Can you work these out from the model? Positions are in its coordinate system, mm. A direction names the side the tool comes from. Round coordinates to 2 decimals unless told otherwise and drop trailing zeros. Loops run counter-clockwise (first coordinate to the right, second up) from the corner with the lowest first, then second, coordinate; pieces in that order, holes last. Notation, with made-up numbers: M 41.25,-29 L 83.25,-29 A17 cw 83.25,-17 Z; hole C -36.5,33.5 d3. An arc over 180 degrees is marked long. Return JSON: item names as keys, results as strings.
Autodesk Inventor part; units mm, degrees
ref_plane "YZ Plane" through (0, 0, 0) normal (1, 0, 0) x (0, 1, 0)
ref_plane "XZ Plane" through (0, 0, 0) normal (0, 1, 0) x (-1, 0, 0)
ref_plane "XY Plane" through (0, 0, 0) normal (0, 0, 1) x (1, 0, 0)
sketch "Sketch1" plane through (0, 0, 0) normal (0, 0, 1) x (1, 0, 0)
  circle A0 centre (0, 0) radius 7
  line L0 (0, 0) -> (0, -11.43) construction
  line L1 (0, -11.43) -> (-50.8, -11.43) construction
  circle A1 centre (-50.8, -11.43) radius 7
  line L2 (0, -11.43) -> (0, -24.13) construction
  line L3 (-50.8, -11.43) -> (-50.8, -24.13) construction
  line L4 (0, -24.13) -> (-101.6, -24.13) construction
  line L5 (-101.6, -24.13) -> (-101.6, -125.73) construction
  line L6 (0, -24.13) -> (12.7, -24.13) construction
  line L7 (-101.6, -125.73) -> (-35.3, -24.13) construction
  line L8 (-101.6, -125.73) -> (15.6852, -125.73) construction
  line L9 (-35.3, -24.13) -> (-117.1955, 29.3117) construction
  line L10 (-117.1955, 29.3117) -> (-143.4272, -10.8866) construction
  line L11 (-123.0577, 33.1371) -> (-149.2895, -7.0611) construction
  line L12 (-137.565, -14.712) -> (-111.3333, 25.4862) construction
  arc A2 (-111.3333, 25.4862) -> (-123.0577, 33.1371) centre (-117.1955, 29.3117) ccw construction
  arc A3 (-149.2895, -7.0611) -> (-137.565, -14.712) centre (-143.4272, -10.8866) ccw construction
  circle A4 centre (-117.1955, 29.3117) radius 12.7 construction
  circle A5 centre (0, 0) radius 120.8055 construction
  circle A6 centre (-50.8, -11.43) radius 92.6288 construction
  line L13 (-101.6, -125.73) -> (-152.4, -125.73) construction
  line L14 (-152.4, -125.73) -> (-152.4, -87.63) construction
  circle A7 centre (-152.4, -87.63) radius 38.1
  line L15 (-152.4, -87.63) -> (-152.4, -49.53) construction
  line L16 (-152.4, -49.53) -> (-152.4, -36.83) construction
  circle A8 centre (-152.4, -36.83) radius 12.7 construction
  circle A9 centre (-117.1955, 29.3117) radius 10.16
  circle A10 centre (-152.4, -36.83) radius 12.7
  line L17 (-163.4022, -30.4863) -> (-125.9972, 34.3866)
  line L18 (-152.4, -49.53) -> (-117.1955, -49.53)
  circle A11 centre (-130.3114, 9.2125) radius 2.05
  circle A12 centre (-143.4272, -10.8866) radius 2.05
  circle A13 centre (-117.1955, 29.3117) radius 7
  circle A14 centre (-152.4, -36.83) radius 7
  line L19 (-117.1955, -49.53) -> (-107.1202, 28.0024)
  point P0 (-152.4, -49.53)
  dimension "d0" = 14
  dimension "d1" = 11.43
  dimension "d2" = 50.8
  dimension "d3" = 14
  dimension "d4" = 12.7
  dimension "d5" = 12.7
  dimension "d6" = 101.6
  dimension "d7" = 101.6
  dimension "d8" = 12.7
  dimension "d9" = 48
  dimension "d14" = 97.79
  dimension "d15" = 90
  dimension "d16" = 48
  dimension "d17" = 14
  dimension "d18" = 25.4
  dimension "d19" = 50.8
  dimension "d20" = 38.1
  dimension "d21" = 12.7
  dimension "d22" = 20.32
  dimension "d24" = 4.1
  dimension "d25" = 4.1
  dimension "d26" = 14
extrude "Extrusion1" add sketch "Sketch1" along normal blind 6.35 contours A10 | A10 L17 A9 L19 L18 | A9
fillet "Fillet1" radius 6.35 1 edges at (-117.1955, -49.53, 3.175)
sketch "Sketch2" plane through (0, 0, 6.35) normal (0, 0, 1) x (1, 0, 0)
  circle A0 centre (-152.4, -36.83) radius 7 construction
  circle A1 centre (-152.4, -36.83) radius 12.7
  circle A2 centre (-117.1955, 29.3117) radius 7 construction
  circle A3 centre (-117.1955, 29.3117) radius 10.16
  line L0 (-125.9972, 34.3866) -> (-163.4022, -30.4863) construction
  arc A4 (-122.7737, -49.53) -> (-116.4767, -43.9983) centre (-122.7737, -43.18) ccw construction
  line L1 (-152.4, -49.53) -> (-122.7737, -49.53) construction
  line L2 (-116.4767, -43.9983) -> (-107.1202, 28.0024) construction
  line L3 (-122.7737, -43.18) -> (-114.631, 19.4806)
  line L4 (-122.7737, -43.18) -> (-149.4542, -43.18)
  circle A5 centre (-143.4272, -10.8866) radius 2.05
  line L5 (-143.4272, -10.8866) -> (-130.3114, 7.1625) construction
  circle A6 centre (-130.3114, 9.2125) radius 2.05
  line L6 (-145.2764, -26.316) -> (-115.2046, 15.0667)
  line L7 (-136.4387, 11.6152) -> (-149.5546, -6.434)
  arc A7 (-149.5546, -6.434) -> (-137.2998, -15.3392) centre (-143.4272, -10.8866) ccw
  arc A8 (-124.184, 2.7099) -> (-136.4387, 11.6152) centre (-130.3114, 7.1625) ccw
  line L8 (-122.7737, -43.18) -> (-137.2998, -15.3392) construction
  line L9 (-119.9588, -41.7113) -> (-134.485, -13.8705)
  line L10 (-140.1147, -16.8079) -> (-125.5886, -44.6487)
  arc A9 (-125.5886, -44.6487) -> (-119.9588, -41.7113) centre (-122.7737, -43.18) ccw
  arc A10 (-134.485, -13.8705) -> (-140.1147, -16.8079) centre (-137.2998, -15.3392) ccw
  point P0 (0, 0)
  point P1 (-136.8693, -1.862)
  point P2 (-130.0368, -29.2596)
  point P3 (-135.4334, -12.7707)
  point P4 (-122.0596, -37.6849)
  point P5 (-126.3549, -43.18)
  point P6 (-139.3843, -18.2077)
  point P7 (-141.4015, -43.18)
  dimension "d30" = 6.35
extrude "Extrusion2" cut sketch "Sketch2" against normal through all contours A1 L6 L10 L4 | L6 L3 L9 A10
fillet "Fillet2" radius 3.175 7 edges at (-115.2046, 15.0667, 3.175) (-122.0596, -37.6849, 3.175) (-135.4334, -12.7707, 3.175) (-139.3843, -18.2077, 3.175) (-126.3549, -43.18, 3.175) (-141.4015, -43.18, 3.175) (-145.2764, -26.316, 3.175)
properties part number "Intake_FourBar_Plate"
Q1. Suppose I cut it at B-B, the plane y = -18.5. Please give me the cut outline in (x, z), plus the area to 3 significant figures.
Results:
{"outline": "M -156.49,0 L -132.07,0 L -132.07,6.35 L -156.49,6.35 Z; M -119.57,0 L -113.16,0 L -113.16,6.35 L -119.57,6.35 Z", "area": "196 mm2"}
Q2. On a 3-axis mill with a long thin cutter (end or side, diameter ignored), from which of +Z, -Z, +X, -X, +Y, -Y can I reach the whole of each face in a straight line? I mean faces 1 (the cylindrical face through (-118.63, -47.99, 3.22)), 2 (the cylindrical face through (-144.144, -26.056, 3.131)). Say none if no direction works.
Results:
{"face 1": "+Z, -Z, +X, -Y", "face 2": "+Z, -Z"}
Q3. Thinking about a two-plate mould opening in Y: for faces 3 (the flat face through (-130.462, -21.582, 3.219)), 4 (the flat face through (-136, -14, 6.35)), 5 (the flat face through (-111.864, -8.502, 3.131)), which applies, pulls with the +Y half, pulls with the -Y half, needs draft (parallel to the pull), parting line crosses it, or undercut?
Results:
{"face 3": "undercut", "face 4": "needs draft", "face 5": "pulls with the -Y half"}
Q4. I'm going to push flat-ended pins straight in: pin 1 Ø1 at (x, z) = (-155, 5.5) entering from -Y; pin 2 Ø1.5 at (y, z) = (-40.5, 1.5) entering from +X. Where does each tip first touch, or does it pass through?
Results:
{"pin 1": "stops at y = -49.36", "pin 2": "stops at x = -115.92"}
Q5. If I drill on line 1 along X through (y, z) = (-33, 5.75); line 2 along Y through (x, z) = (-130, 1.75); line 3 along Y through (x, z) = (-129.5, 4.75), over which ranges is the centre line in solid material (lowest first)?
Results:
{"line 1": "x = -164.51 to -158.26, -146.54 to -140.29, -131.67 to -115.05", "line 2": "y = -49.53 to -42.75, -36.19 to -22.47, -5.29 to 7.19, 11.24 to 27.44", "line 3": "y = -49.53 to -42.39, -37.15 to -23.42, -4.61 to 7.33, 11.1 to 28.31"}
Q6. Suppose I cut it at C-C, the plane y = -36.83. Please give me the cut outline in (x, z), plus the area to 3 significant figures.
Results:
{"outline": "M -165.1,0 L -159.4,0 L -159.4,6.35 L -165.1,6.35 Z; M -145.4,0 L -139.7,0 L -139.7,6.35 L -145.4,6.35 Z; M -129.67,0 L -115.55,0 L -115.55,6.35 L -129.67,6.35 Z", "area": "162 mm2"}
Q7. Suppose I cut it at D-D, the plane z = 3.5. State how many separate pieces and enclosed holes the cut face has, plus the area to 3 significant figures.
Results:
{"separate pieces": "1", "enclosed holes": "6", "area": "2,250 mm2"}
Q8. Suppose I cut it at A-A, the plane x = -138. Please give me the cut outline in (y, z), plus the area to 3 significant figures.
Results:
{"outline": "M -49.53,0 L -42.96,0 L -42.96,6.35 L -49.53,6.35 Z; M -21.62,0 L 13.57,0 L 13.57,6.35 L -21.62,6.35 Z", "area": "265 mm2"}
